Can you work these out from the model? Positions are in its coordinate system, mm. Face numbers are marked on the shaded views. Round coordinates to 2 decimals unless told otherwise and drop trailing zeros. Loops run counter-clockwise (first coordinate to the right, second up) from the corner with the lowest first, then second, coordinate; pieces in that order, holes last. Notation, with made-up numbers: M 58.25,24 L 110.25,24 A12 cw 110.25,34 Z; hole C 89.5,-33 d8. An arc over 180 degrees is marked long. Answer as CSV lines item,"result".
from build123d import *

# Parameters (mm, degrees)
SKETCH_1_R      = 12.5
SKETCH_1_R_2    = 9
EXTRUDE_1_DEPTH = 6.3
SKETCH_2_R      = 13.5
SKETCH_2_R_2    = 9
EXTRUDE_2_DEPTH = 5.8
SKETCH_3_W      = 46
SKETCH_3_H      = 24
SKETCH_3_R      = 9
SKETCH_3_R_2    = 1.6
EXTRUDE_3_DEPTH = 2
FILLET_1_R      = 3
EXTRUDE_4_DEPTH = 2


with BuildPart() as part:
    # 草图1 → 凸台-拉伸1 (new body)
    with BuildSketch(Plane.XY):
        Circle(SKETCH_1_R)
        Circle(SKETCH_1_R_2, mode=Mode.SUBTRACT)
    extrude(amount=EXTRUDE_1_DEPTH)

    # 草图2 → 凸台-拉伸2 (add)
    with BuildSketch(Plane.XY.offset(6.3)):
        Circle(SKETCH_2_R)
        Circle(SKETCH_2_R_2, mode=Mode.SUBTRACT)
    extrude(amount=EXTRUDE_2_DEPTH)

    # 草图3 → 凸台-拉伸3 (add)
    with BuildSketch(Plane.XY.offset(12.1)):
        Rectangle(SKETCH_3_W, SKETCH_3_H)
        Circle(SKETCH_3_R, mode=Mode.SUBTRACT)
        with Locations((18, 8)):
            Circle(SKETCH_3_R_2, mode=Mode.SUBTRACT)
        with Locations(Location((18, -8, 0), (0, 0, 180))):
            Circle(SKETCH_3_R_2, mode=Mode.SUBTRACT)
        with Locations((-18, -8)):
            Circle(SKETCH_3_R_2, mode=Mode.SUBTRACT)
        with Locations(Location((-18, 8, 0), (0, 0, 180))):
            Circle(SKETCH_3_R_2, mode=Mode.SUBTRACT)
    extrude(amount=EXTRUDE_3_DEPTH)

    # 圆角1
    fillet_1_edges = [part.edges().sort_by_distance(p)[0] for p in [
        (23, 12, 13.1),
        (-23, 12, 13.1),
        (-23, -12, 13.1),
        (23, -12, 13.1),
    ]]
    fillet(fillet_1_edges, radius=FILLET_1_R)

    # 草图4 → 凸台-拉伸4 (add)
    with BuildSketch(Plane.XY.offset(12.1)):
        with BuildLine():
            Line((6.184658438, -12), (-6.184658438, -12))
            ThreePointArc((-6.184658438, -12), (0, -13.5), (6.184658438, -12))
        make_face()
        with BuildLine():
            Line((-6.184658438, 12), (6.184658438, 12))
            ThreePointArc((6.184658438, 12), (0, 13.5), (-6.184658438, 12))
        make_face()
    extrude(amount=EXTRUDE_4_DEPTH)


solid = part.part
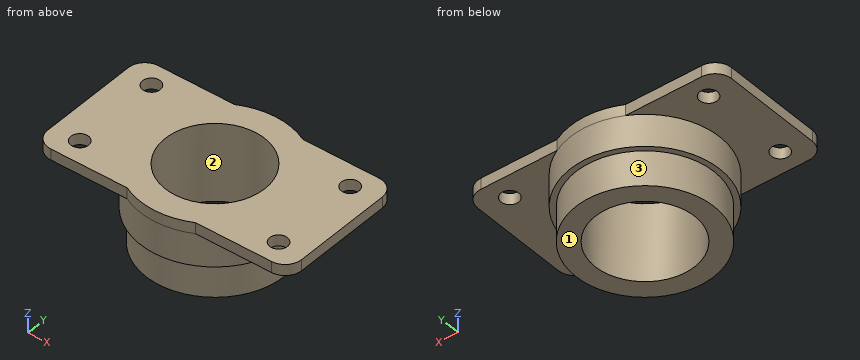
Item 1: If I drill on line 1 along Y through (x, z) = (18, 13.35); line 2 along Y through (x, z) = (0, 6.5); line 3 along Z through (x, y) = (15, 8.25), over which ranges is the centre line in solid material (lowest first)? Write a range as from..to.
Output:
line 1,"y = -12..-9.6, -6.4..6.4, 9.6..12"
line 2,"y = -13.5..-9, 9..13.5"
line 3,"z = 12.1..14.1"
Item 2: If we section it at D-D on z = 1.75: Write out the boundary of the cut face in (x, y), then the cut area to 3 significant figures.
Output:
outline,"C 0,0 d25; hole C 0,0 d18"
area,"236 mm2"
Item 3: If we section it at B-B on y = 0: Write out the boundary of the cut face in (x, z), then the cut area to 3 significant figures.
Output:
outline,"M -23,12.1 L -13.5,12.1 L -13.5,6.3 L -12.5,6.3 L -12.5,0 L -9,0 L -9,14.1 L -23,14.1 Z; M 9,0 L 12.5,0 L 12.5,6.3 L 13.5,6.3 L 13.5,12.1 L 23,12.1 L 23,14.1 L 9,14.1 Z"
area,"152 mm2"
Item 4: If we section it at C-C on x = 0: Write out the boundary of the cut face in (y, z), then the cut area to 3 significant figures.
Output:
outline,"M -13.5,6.3 L -12.5,6.3 L -12.5,0 L -9,0 L -9,14.1 L -13.5,14.1 Z; M 9,0 L 12.5,0 L 12.5,6.3 L 13.5,6.3 L 13.5,14.1 L 9,14.1 Z"
area,"114 mm2"
Item 5: We'd pull the mould along X, two halves only. Please class the marked faces 1, 2 and 3: released by +X, released by -X, zero draft, split by the parting line, or undercut.
Output:
face 1,"zero draft"
face 2,"undercut"
face 3,"split by the parting line"
Item 6: If we section it at A-A on x = -18: Write out the boundary of the cut face in (y, z).
Output:
outline,"M -12,12.1 L -9.6,12.1 L -9.6,14.1 L -12,14.1 Z; M -6.4,12.1 L 6.4,12.1 L 6.4,14.1 L -6.4,14.1 Z; M 9.6,12.1 L 12,12.1 L 12,14.1 L 9.6,14.1 Z"
Item 7: Will these pins go through, and if not, where does the flat tip stop? pin 1 (1 mm diameter, centred on x = 10, z = 13.5, fed in from -Y); pin 2 (2 mm diameter, centred on y = 5, z = 3.5, fed in from +X); pin 3 (2 mm diameter, centred on x = 10.5, z = 13.5, fed in from +Y).
Output:
pin 1,"stops at y = -12"
pin 2,"stops at x = 11.84"
pin 3,"stops at y = 12"
